Source: three-view drawing plus pictorial views. Frame: mm from the lowest corner of the part. Give positions to 0.01 mm unless a question says otherwise; leave off trailing zeros. Write each loop counter-clockwise with the first axis right and the second up, starting at its lowest first coordinate (ties: lowest second). Pieces come first, ordered by that corner, then holes. Notation, with made-up numbers: (9.25, 61.5) -> (16.25, 61.5) arc R14 cw to (16.25, 77.5) -> close; hole circle Ø2 at (37, 10). An arc over 180 degrees is marked (long way). Write item = value, one per line.
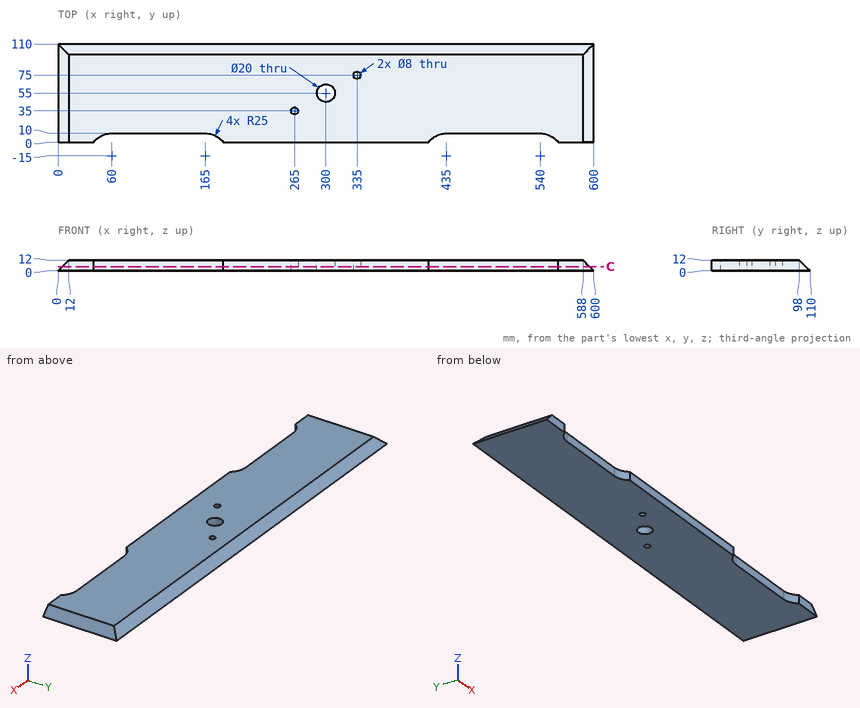
1) Material intervals for L1, parallel to X at y = 5, z = 11.25; L2, parallel to X at y = 49, z = 4.5; L3, parallel to Y at x = 265, z = 6.5, sorted ascending.
Computed:
L1 = 11.25 to 45, 180 to 420, 555 to 588.75
L2 = 4.5 to 292, 308 to 595.5
L3 = 0 to 31, 39 to 103.5
2) Cut plane C-C (z = 4.75). Return the cut outline in (x, y).
Computed:
outline = (4.75, 0) -> (40, 0) arc R25 cw to (60, 10) -> (165, 10) arc R25 cw to (185, 0) -> (415, 0) arc R25 cw to (435, 10) -> (540, 10) arc R25 cw to (560, 0) -> (595.25, 0) -> (595.25, 105.25) -> (4.75, 105.25) -> close; hole circle Ø8 at (265, 35); hole circle Ø20 at (300, 55); hole circle Ø8 at (335, 75)
3) Contact query for flat-ended pins moving along their axis: pin 1 (3 mm diameter, centred on x = 492.5, z = 7, fed in from +Y); pin 2 (4 mm diameter, centred on x = 290.5, z = 11, fed in from +Y); pin 3 (5 mm diameter, centred on y = 52.5, z = 3.5, fed in from -X). Output: stop coordinate, or through.
Computed:
pin_1 = 104.5
pin_2 = 101
pin_3 = 1
